The listing builds one solid part. Answer for the finished solid, in the listing's coordinates (mm). Face numbers are marked on the shaded views. A direction names the side the tool comes from. Coordinates: 2 decimals unless noted, no trailing zeros. Loops run counter-clockwise (first coordinate to the right, second up) from the corner with the lowest first, then second, coordinate; pieces in that order, holes last. Notation, with made-up numbers: (56.25, 85) - (87.25, 85) arc R19 cw to (87.25, 89) - close; hole circle Ø3 at (-20, 62.5). An arc over 180 degrees is marked (long way). One line per question, with ' | ' between items.
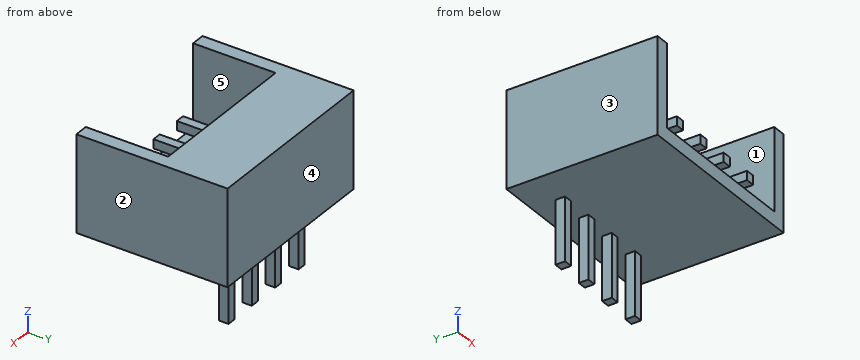
from build123d import *

# Parameters (mm, degrees)
SKETCH_1_W                 = 6.75
SKETCH_1_H                 = 5.5
EXTRUDE_1_DEPTH            = 3.5
SKETCH_2_W                 = 0.32
SKETCH_2_H                 = 0.35
EXTRUDE_2_DEPTH            = 2.3
SKETCH_3_W                 = 5.75
SKETCH_3_H                 = 3
CUT_EXTRUDE_1_DEPTH        = 3
SKETCH_4_W                 = 0.33
SKETCH_4_H                 = 0.33
EXTRUDE_3_DEPTH            = 2.8
PATTERN_LINEAR_3_COUNT     = 2
PATTERN_LINEAR_3_PITCH     = 1.25
PATTERN_LINEAR_3_COL_COUNT = 3
PATTERN_LINEAR_3_COL_PITCH = 1.25


with BuildPart() as part:
    # Эскиз1 → Бобышка-Вытянуть1 (new body)
    with BuildSketch(Plane.XY):
        with Locations((0, 2.75)):
            Rectangle(SKETCH_1_W, SKETCH_1_H)
    extrude(amount=EXTRUDE_1_DEPTH)

    # Эскиз2 → Бобышка-Вытянуть2 (add)
    with BuildSketch(Plane(origin=(0, 0, 0), x_dir=(-1, 0, 0), z_dir=(0, 0, -1))):
        with Locations((-0.625, 4.45)):
            Rectangle(SKETCH_2_W, SKETCH_2_H)
    extrude_2 = extrude(amount=EXTRUDE_2_DEPTH)

    # Эскиз3 → Вырез-Вытянуть1 (cut)
    with BuildSketch(Plane.XZ):
        with Locations((0, 2)):
            Rectangle(SKETCH_3_W, SKETCH_3_H)
    extrude(amount=-CUT_EXTRUDE_1_DEPTH, mode=Mode.SUBTRACT)

    # Эскиз4 → Бобышка-Вытянуть3 (add)
    with BuildSketch(Plane.XZ.offset(-3)):
        with Locations((0.625, 1.25)):
            Rectangle(SKETCH_4_W, SKETCH_4_H)
    extrude_3 = extrude(amount=EXTRUDE_3_DEPTH)

    # Линейный массив3: Бобышка-Вытянуть2, Бобышка-Вытянуть3 ×2
    with Locations(*[(i * PATTERN_LINEAR_3_PITCH, 0, 0) for i in range(1, PATTERN_LINEAR_3_COUNT)]):
        add(extrude_2)
        add(extrude_3)

    # Линейный массив3 col: Бобышка-Вытянуть2, Бобышка-Вытянуть3 ×3
    with Locations(*[(-i * PATTERN_LINEAR_3_COL_PITCH, 0, 0) for i in range(1, PATTERN_LINEAR_3_COL_COUNT)]):
        add(extrude_2)
        add(extrude_3)


solid = part.part
Item 1: Find section C-C, the plane z = 3. Write down the section's boundary in (x, y) (3 decimals).
Taken from the geometry:
outline: (-3.375, 0) - (-2.875, 0) - (-2.875, 3) - (2.875, 3) - (2.875, 0) - (3.375, 0) - (3.375, 5.5) - (-3.375, 5.5) - close
Item 2: Find the intervals of material crossed by line 1 (X direction, y = 4.35, z = -0.4) (3 decimals); line 2 (X direction, y = 2.4, z = 2.6) (3 decimals); line 3 (Z direction, x = 0, y = 2.05), in increasing order. Write a range as [from, to].
Taken from the geometry:
line 1: x = [-2.035, -1.715], [-0.785, -0.465], [0.465, 0.785], [1.715, 2.035] | line 2: x = [-3.375, -2.875], [2.875, 3.375] | line 3: z = [0, 0.5]
Item 3: Find section A-A, the plane z = -0.4. Write down the section's boundary in (x, y) (3 decimals).
Taken from the geometry:
outline: (-2.035, 4.275) - (-1.715, 4.275) - (-1.715, 4.625) - (-2.035, 4.625) - close; (-0.785, 4.275) - (-0.465, 4.275) - (-0.465, 4.625) - (-0.785, 4.625) - close; (0.465, 4.275) - (0.785, 4.275) - (0.785, 4.625) - (0.465, 4.625) - close; (1.715, 4.275) - (2.035, 4.275) - (2.035, 4.625) - (1.715, 4.625) - close
Item 4: Find section D-D, the plane x = 2.5. Write down the section's boundary in (y, z), plus the area to 4 significant figures.
Taken from the geometry:
outline: (0, 0) - (5.5, 0) - (5.5, 3.5) - (3, 3.5) - (3, 0.5) - (0, 0.5) - close | area: 10.25 mm2
Item 5: This flat-tipped pin is pushed along its axis until it touches: pin 1 Ø2 at (x, y) = (2.5, 1) entering from +Z. Where does it stop, or does it pass through?
Taken from the geometry:
pin 1: stops at z = 3.5
Item 6: Find section B-B, the plane y = 1.7. Write down the section's boundary in (x, z) (3 decimals), plus the area to 3 significant figures.
Taken from the geometry:
outline: (-3.375, 0) - (3.375, 0) - (3.375, 3.5) - (2.875, 3.5) - (2.875, 0.5) - (-2.875, 0.5) - (-2.875, 3.5) - (-3.375, 3.5) - close; (-2.04, 1.085) - (-1.71, 1.085) - (-1.71, 1.415) - (-2.04, 1.415) - close; (-0.79, 1.085) - (-0.46, 1.085) - (-0.46, 1.415) - (-0.79, 1.415) - close; (0.46, 1.085) - (0.79, 1.085) - (0.79, 1.415) - (0.46, 1.415) - close; (1.71, 1.085) - (2.04, 1.085) - (2.04, 1.415) - (1.71, 1.415) - close | area: 6.81 mm2
Item 7: Which of the six approach directions +Z, -Z, +X, -X, +Y, -Y give full straight-line access (tool end or side, diameter ignored) to the marked faces 1 and 2?
Taken from the geometry:
face 1: +Z, -Y | face 2: +Z, -Z, +X, +Y, -Y
Item 8: The mould has two halves that part along X. Classify the marked faces 3, 4 and 5: pulls with the +X half, pulls with the -X half, needs draft (parallel to the pull), parting line crosses it, or undercut.
Taken from the geometry:
face 3: pulls with the -X half | face 4: needs draft | face 5: undercut
